Study the drawing (mm; zero at the part's minimum x, y, z) and answer. A direction names the side the tool comes from. Coordinates: 2 decimals unless noted, no trailing zeros.
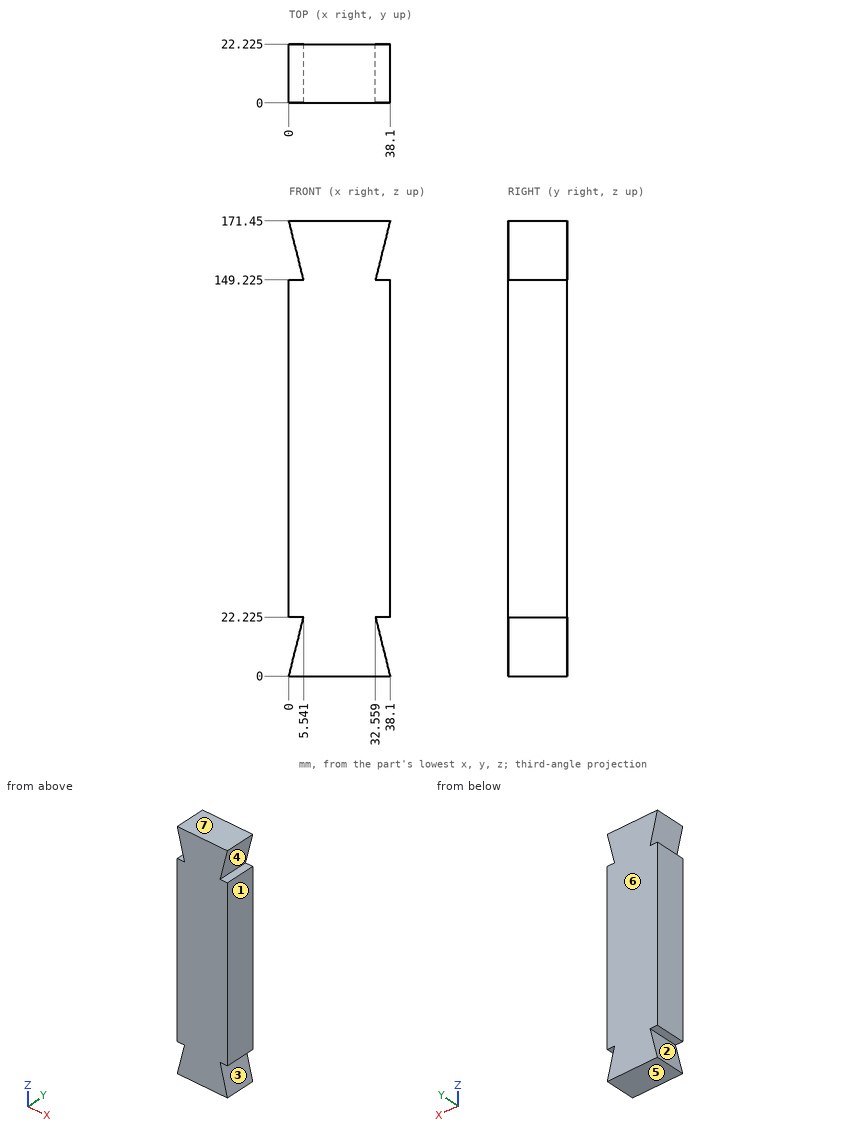
(1) Given pin 1 Ø8 at (y, z) = (12.5, 152) entering from +X, flat-ended and moving along its own axis, determine where the tip first touches the part or whether it passes through.
(2) The mould has two halves that part along Z. Classify the marked faces 4, 5, 6 and 7: pulls with the +Z half, pulls with the -Z half, needs draft (parallel to the pull), parting line crosses it, or undercut.
(3) Find the intervals of material crossed by probe 1 along X at (y, z) = (16, 15.5) (1 decimal); probe 2 along X at (y, z) = (7.5, 19.5), in increasing order.
(4) A tool of negligible diameter and unlimited length cuts with its end or side. For the marked faces 1, 2 and 3, from which of +Z, -Z, +X, -X, +Y, -Y can it reach the whole face along a straight path? Write none if from no direction.
Resolved:
1. pin 1: stops at x = 38.1
2. face 4: undercut
2. face 5: pulls with the -Z half
2. face 6: needs draft
2. face 7: pulls with the +Z half
3. probe 1: x = 3.9 to 34.2
3. probe 2: x = 4.86 to 33.24
4. face 1: +Z, -Z, +X, +Y, -Y
4. face 2: -X, +Y, -Y
4. face 3: +X, +Y, -Y
